The listing builds one solid part. Answer for the finished solid, in the listing's coordinates (mm). Coordinates: 2 decimals unless noted, no trailing zeros. Write each loop counter-clockwise with the first axis right and the second up, starting at its lowest first coordinate (ties: lowest second). Pieces come first, ordered by that corner, then holes. Notation, with made-up numbers: M 30.5,44.25 L 68.5,44.25 A21 ccw 68.5,56.25 Z; hole C -13.75,35 d2. An arc over 180 degrees is marked long. Answer as CSV lines item,"result". Start each with the question number.
Autodesk Inventor part; units mm, degrees
ref_plane "YZ Plane" through (0, 0, 0) normal (1, 0, 0) x (0, 1, 0)
ref_plane "XZ Plane" through (0, 0, 0) normal (0, 1, 0) x (-1, 0, 0)
ref_plane "XY Plane" through (0, 0, 0) normal (0, 0, 1) x (1, 0, 0)
sketch "Sketch1" plane through (0, 0, 0) normal (0, 0, 1) x (1, 0, 0)
  line L0 (-12.7, -31.75) -> (12.7, -31.75)
  line L1 (12.7, -31.75) -> (12.7, 31.75)
  line L2 (12.7, 31.75) -> (-12.7, 31.75)
  line L3 (-12.7, 31.75) -> (-12.7, -31.75)
  line L4 (-12.7, -31.75) -> (12.7, 31.75) construction
  line L5 (12.7, -31.75) -> (-12.7, 31.75) construction
  point P0 (0, 0)
  dimension "d0" = 25.4
  dimension "d1" = 63.5
extrude "Extrusion1" add sketch "Sketch1" along normal blind 12.7
sketch "Sketch2" plane through (0, 0, 12.7) normal (0, 0, 1) x (1, 0, 0)
  line L0 (-12.7, -31.75) -> (12.7, -31.75)
  line L1 (12.7, 31.75) -> (-12.7, 31.75)
  line L2 (-12.7, 31.75) -> (-12.7, -31.75)
  line L3 (0, 31.75) -> (0, 25.4)
  line L4 (0, -31.75) -> (0, -25.4)
  point P0 (0, 0)
  dimension "d4" = 6.35
  dimension "d5" = 6.35
hole "Hole2" at (0, 25.4, 12.7) at (0, -25.4, 12.7) direction (0, 0, -1) diameter 6.35 end through all
sketch "Sketch3" plane through (0, 0, 12.7) normal (0, 0, 1) x (1, 0, 0)
  point P0 (0, 0)
hole "Hole3" at (0, 0, 12.7) direction (0, 0, -1) diameter 12.7 end through all
properties part number "3 in bar"
1) The part is cut by section B-B (x = 0). Determine the outline of the cut face in (y, z) (3 decimals), then the cut area to 3 significant figures.
2) Find the intervals of material crossed by line 1 (Y direction, x = 1.5, z = 6.5); line 2 (Y direction, x = 0, z = 4.25) (3 decimals); line 3 (X direction, y = 25.4, z = 10) (3 decimals), in increasing order. Write a range as from..to.
3) This flat-tipped pin is pushed along its axis until it touches: P1, Ø5.5, axis at x = 0, y = -25.4, coming from the +Z side. Where does it stop, or does it pass through?
4) The part is cut by section A-A (z = 10.5). Determine the outline of the cut face in (x, y) (3 decimals), then the cut area to 3 significant figures.
5) For a pull along Y with two mould halves and no side action, classify faces 1 (the face through (6.2, 1.38, 6.26)), 2 (the face through (0, 31.75, 6)), 3 (the face through (0, 8, 12.7)) as +Y half, -Y half, draft (parallel to the pull), parting line (faces both ways), or undercut.
6) The part is cut by section C-C (y = -25.4). Determine the outline of the cut face in (x, z) (3 decimals), then the cut area to 3 significant figures.
7) The part is cut by section D-D (x = 5.5). Determine the outline of the cut face in (y, z), then the cut area to 3 significant figures.
Completed:
1,outline,"M -31.75,0 L -28.575,0 L -28.575,12.7 L -31.75,12.7 Z; M -22.225,0 L -6.35,0 L -6.35,12.7 L -22.225,12.7 Z; M 6.35,0 L 22.225,0 L 22.225,12.7 L 6.35,12.7 Z; M 28.575,0 L 31.75,0 L 31.75,12.7 L 28.575,12.7 Z"
1,area,"484 mm²"
2,line 1,"-31.75..-28.2, -22.6..-6.17, 6.17..22.6, 28.2..31.75"
2,line 2,"-31.75..-28.575, -22.225..-6.35, 6.35..22.225, 28.575..31.75"
2,line 3,"-12.7..-3.175, 3.175..12.7"
3,P1,"through"
4,outline,"M -12.7,-31.75 L 12.7,-31.75 L 12.7,31.75 L -12.7,31.75 Z; hole C 0,0 d12.7; hole C 0,-25.4 d6.35; hole C 0,25.4 d6.35"
4,area,"1,420 mm²"
5,face 1,"undercut"
5,face 2,"+Y half"
5,face 3,"draft"
6,outline,"M -12.7,0 L -3.175,0 L -3.175,12.7 L -12.7,12.7 Z; M 3.175,0 L 12.7,0 L 12.7,12.7 L 3.175,12.7 Z"
6,area,"242 mm²"
7,outline,"M -31.75,0 L -3.17,0 L -3.17,12.7 L -31.75,12.7 Z; M 3.17,0 L 31.75,0 L 31.75,12.7 L 3.17,12.7 Z"
7,area,"726 mm²"
